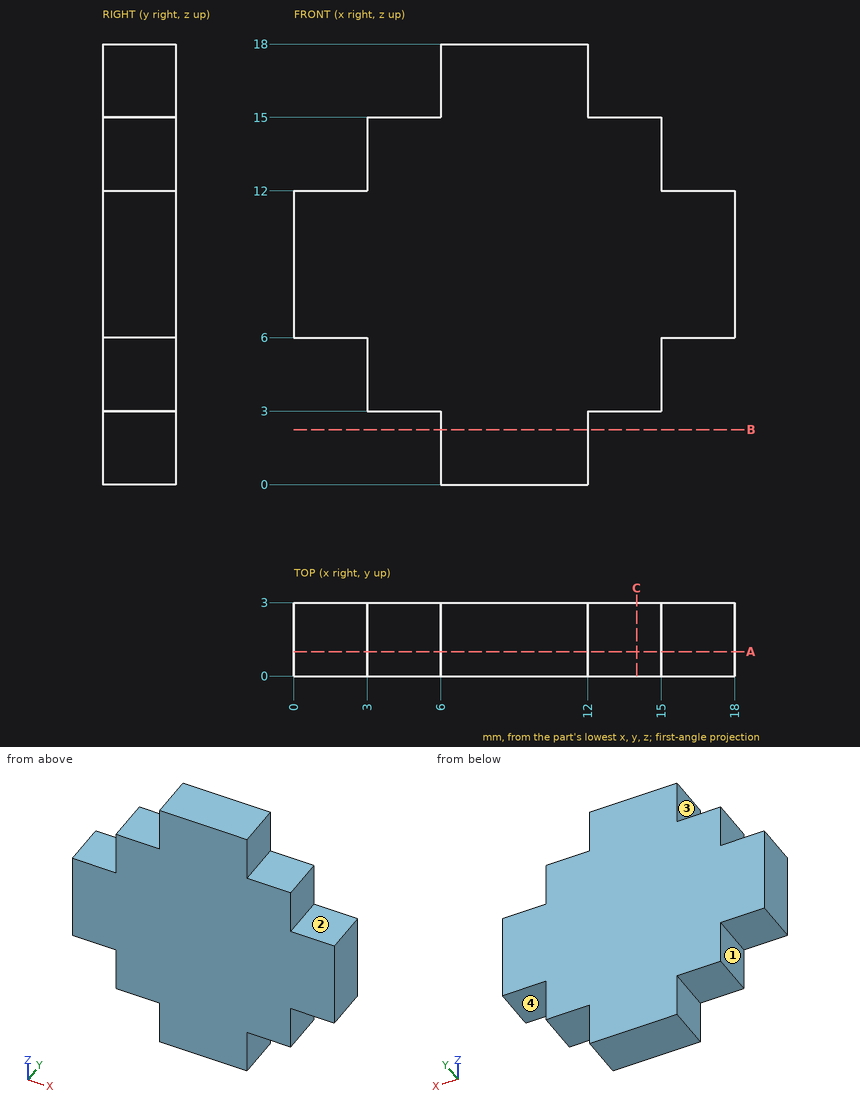
Check sheet for the drawn part. Datum: minimum x, y, z corner. Units: mm. A direction names the side the tool comes from. Give positions to 0.01 mm unless a question says otherwise; leave off trailing zeros. Write each loop counter-clockwise with the first axis right and the second up, starting at its lowest first coordinate (ties: lowest second). Pieces come first, ordered by that corner, then holes. Notation, with made-up numbers: (39, 46) - (72, 46) arc R4 cw to (72, 51) - close; hole circle Ø5 at (7, -2.5). An arc over 180 degrees is marked (long way). Put each result on its own line as item: value.
1. Thickness scan on line 1 (Z direction, x = 12.75, y = 2.35); line 2 (X direction, y = 1.8, z = 2.75). Record the ranges inside material, lowest first.
Ans:
line 1: z = 3 to 15
line 2: x = 6 to 12
2. Go/stop test with flat-tipped pins: pin 1 (1.5 mm diameter, centred on x = 3.5, y = 2.5, fed in from +Z); pin 2 (10 mm diameter, centred on x = 6, z = 5, fed in from -Y); pin 3 (1 mm diameter, centred on x = 5, y = 1.5, fed in from -Z); pin 4 (1.5 mm diameter, centred on y = 1.5, z = 17, fed in from +X). Record where each tip stops, or that it passes through.
Ans:
pin 1: stops at z = 15
pin 2: stops at y = 0
pin 3: stops at z = 3
pin 4: stops at x = 12
3. Sectioned sample at C-C, the plane x = 14. Enter the section's corners in (y, z).
Ans:
outline: (0, 3) - (3, 3) - (3, 15) - (0, 15) - close
4. Sectioned sample at A-A, the plane y = 1. Enter the section's corners in (x, z), plus the area to 3 significant figures.
Ans:
outline: (0, 6) - (3, 6) - (3, 3) - (6, 3) - (6, 0) - (12, 0) - (12, 3) - (15, 3) - (15, 6) - (18, 6) - (18, 12) - (15, 12) - (15, 15) - (12, 15) - (12, 18) - (6, 18) - (6, 15) - (3, 15) - (3, 12) - (0, 12) - close
area: 216 mm²
5. Set-up check for the marked faces 1, 2, 3 and 4: record each of +Z, -Z, +X, -X, +Y, -Y from which the full face is reachable in a straight line by a thin tool's end or side.
Ans:
face 1: -Z, -X, +Y, -Y
face 2: +Z, +X, +Y, -Y
face 3: +Z, -X, +Y, -Y
face 4: -Z, +X, +Y, -Y
6. Sectioned sample at B-B, the plane z = 2.25. Enter the section's corners in (x, y).
Ans:
outline: (6, 0) - (12, 0) - (12, 3) - (6, 3) - close
